Can you work these out from the model? Positions are in its coordinate system, mm. A direction names the side the tool comes from. Coordinates: 2 decimals unless noted, no trailing zeros. Loops run counter-clockwise (first coordinate to the right, second up) from the corner with the lowest first, then second, coordinate; pieces in that order, holes last. Notation, with made-up numbers: M 56.5,-33.5 L 83.5,-33.5 A17 cw 83.5,-16.5 Z; hole C 8.5,79 d9. An arc over 180 degrees is marked long. Answer as a JSON object with one key per item and string values. Group by question number.
Item 1: Which directions (+Z, -Z, +X, -X, +Y, -Y) give clear straight access to the entire face, cutting with the end or side of a thin tool? Please do faces 5 (the flat face through (-1.651, 213, 13)), 6 (the flat face through (0, 213, 13)).
Item 2: If I drill on line 1 (Y direction, x = -1, z = 12.7); line 2 (Z direction, x = -26, y = 89); line 3 (X direction, y = 156.5, z = 12), over which ranges is the centre line in solid material (lowest first)?
Item 3: Suppose I cut it at C-C (z = 6). Write out the boundary of the cut face in (x, y), then the cut area to 3 significant figures.
Item 4: Suppose I cut it at A-A (x = -44). Write out the boundary of the cut face in (y, z), then the cut area to 3 significant figures.
Item 5: Suppose I cut it at D-D (x = -25.4). Write out the boundary of the cut face in (y, z) (3 decimals).
Item 6: We'd pull the mould along Y, two halves only. Please class faces 1 (the cylindrical face through (-27.46, 371.7, 0.84)), 2 (the flat face through (-23, 431.8, 1)), 3 (the flat face through (-50.8, 213, 13)), 4 (the cylindrical face through (-27.46, 371.7, 24.59)): +Y half, -Y half, draft (parallel to the pull), parting line (faces both ways), or undercut.
Item 7: Suppose I cut it at B-B (y = 264). Write out the boundary of the cut face in (x, z).
Autodesk Inventor part; units mm, degrees
ref_plane "YZ Plane" through (0, 0, 0) normal (1, 0, 0) x (0, 1, 0)
ref_plane "XZ Plane" through (0, 0, 0) normal (0, 1, 0) x (-1, 0, 0)
ref_plane "XY Plane" through (0, 0, 0) normal (0, 0, 1) x (1, 0, 0)
sketch "Sketch1" plane through (0, 0, 0) normal (0, 1, 0) x (-1, 0, 0)
  line L0 (0, 0) -> (50.8, 0)
  line L1 (50.8, 0) -> (50.8, 25.4)
  line L2 (50.8, 25.4) -> (0, 25.4)
  line L3 (0, 25.4) -> (0, 0)
  line L4 (49.149, 23.749) -> (1.651, 23.749)
  line L5 (1.651, 23.749) -> (1.651, 1.651)
  line L6 (1.651, 1.651) -> (49.149, 1.651)
  line L7 (49.149, 1.651) -> (49.149, 23.749)
  dimension "d0" = 50.8
  dimension "d1" = 25.4
  dimension "d2" = 1.651
  dimension "d3" = 1.651
  dimension "d4" = 1.651
  dimension "d5" = 1.651
extrude "Extrusion1" add sketch "Sketch1" along normal blind 431.8
sketch "Sketch2" plane through (-50.8, 0, 0) normal (-1, 0, 0) x (0, 0, 1)
  circle A0 centre (12.7, 38.1) radius 2.5797
  circle A1 centre (12.7, 63.5) radius 2.5797
  circle A2 centre (12.7, 88.9) radius 2.5797
  line L0 (0, 0) -> (0, 431.8)
  line L1 (0, 0) -> (25.4, 0)
  dimension "d8" = 5.1594
  dimension "d9" = 12.7
  dimension "d10" = 12.7
  dimension "d11" = 12.7
  dimension "d12" = 5.1594
  dimension "d13" = 5.1594
  dimension "d14" = 25.4
  dimension "d15" = 50.8
  dimension "d16" = 38.1
extrude "Extrusion2" cut sketch "Sketch2" against normal blind 609.6
sketch "Sketch3" plane through (-50.8, 0, 25.4) normal (0, 0, 1) x (1, 0, 0)
  circle A0 centre (25.4, 381) radius 9.525
  line L0 (0, 431.8) -> (50.8, 431.8)
  line L1 (50.8, 0) -> (50.8, 431.8)
  dimension "d19" = 19.05
  dimension "d20" = 50.8
  dimension "d26" = 25.4
extrude "Extrusion3" cut sketch "Sketch3" against normal blind 25.4
equation "\"d3\" = d2"
equation "\"d4\" = d2"
equation "\"d5\" = d2"
equation "\"d10\" = d9"
equation "\"d11\" = d9"
equation "\"d12\" = d8"
equation "\"d13\" = d8"
properties part number "mounting part 2"
From the geometry:
{
 "1": {"face 5": "+Y, -Y", "face 6": "+Z, -Z, +X, +Y, -Y"},
 "2": {"line 1": "0 to 35.52, 40.68 to 60.92, 66.08 to 86.32, 91.48 to 431.8", "line 2": "0 to 1.65, 23.75 to 25.4", "line 3": "-50.8 to -49.15, -1.65 to 0"},
 "3": {"outline": "M -50.8,0 L -49.15,0 L -49.15,431.8 L -50.8,431.8 Z; M -1.65,0 L 0,0 L 0,431.8 L -1.65,431.8 Z", "area": "1,430 mm2"},
 "4": {"outline": "M 0,0 L 431.8,0 L 431.8,1.65 L 0,1.65 Z; M 0,23.75 L 431.8,23.75 L 431.8,25.4 L 0,25.4 Z", "area": "1,430 mm2"},
 "5": {"outline": "M 0,0 L 371.475,0 L 371.475,1.651 L 0,1.651 Z; M 0,23.749 L 371.475,23.749 L 371.475,25.4 L 0,25.4 Z; M 390.525,0 L 431.8,0 L 431.8,1.651 L 390.525,1.651 Z; M 390.525,23.749 L 431.8,23.749 L 431.8,25.4 L 390.525,25.4 Z"},
 "6": {"face 1": "undercut", "face 2": "+Y half", "face 3": "draft", "face 4": "undercut"},
 "7": {"outline": "M -50.8,0 L 0,0 L 0,25.4 L -50.8,25.4 Z; hole M -49.15,1.65 L -1.65,1.65 L -1.65,23.75 L -49.15,23.75 Z"}
}
